Geometry check sheet. Reference: the model listing, model coordinates, mm. A direction names the side the tool comes from. Coordinates: 2 decimals unless noted, no trailing zeros. Loops run counter-clockwise (first coordinate to the right, second up) from the corner with the lowest first, then second, coordinate; pieces in that order, holes last.
Autodesk Inventor part; units mm, degrees
ref_plane "Work Plane1" through (0, 0, 0) normal (0, 0, 1) x (1, 0, 0)
ref_plane "Work Plane2" through (0, 0, 0) normal (0, 0, 1) x (1, 0, 0)
ref_plane "YZ Plane" through (0, 0, 0) normal (1, 0, 0) x (0, 1, 0)
ref_plane "Work Plane1" through (0, 0, 0) normal (0, 0, 1) x (1, 0, 0)
sketch "Sketch1" plane through (0, 0, 0) normal (0, 0, 1) x (1, 0, 0)
  circle A0 centre (0, -92.5) radius 4
  circle A1 centre (0, -102.5) radius 1.5
  circle A2 centre (-10, -92.5) radius 1.5
  circle A3 centre (0, -82.5) radius 1.5
  circle A4 centre (10, -92.5) radius 1.5
  circle A5 centre (0, -92.5) radius 13
  circle A6 centre (0, -92.5) radius 7
  point P0 (0, 0)
  dimension "d0" = 26
  dimension "d1" = 14
extrude "Extrusion1" add sketch "Sketch1" along normal blind 2 contours A5
ref_plane "Work Plane2" through (0, 0, 0) normal (0, 0, 1) x (1, 0, 0)
sketch "Sketch2" plane through (0, 0, 0) normal (0, 0, 1) x (1, 0, 0)
  circle A0 centre (0, -92.5) radius 7
  circle A1 centre (0, -92.5) radius 4
  point P0 (0, 0)
extrude "Extrusion2" add sketch "Sketch2" along normal blind 12
properties part number "AcopleBrida8mm" material "Aluminio 6061"
(1) Sectioned sample at C-C on z = 1. Record the cut outline in (x, y).
Findings:
outline: circle Ø26 at (0, -92.5); hole circle Ø3 at (-10, -92.5); hole circle Ø8 at (0, -92.5); hole circle Ø3 at (0, -102.5); hole circle Ø3 at (0, -82.5); hole circle Ø3 at (10, -92.5)
(2) Gauge pin test, flat ends, axial feed: pin 1 Ø3 at (x, z) = (-5, 9.5) entering from +Y; pin 2 Ø4 at (x, y) = (10, -92.5) entering from +Z; pin 3 Ø3 at (x, z) = (-6, 9) entering from +Y; pin 4 Ø2.5 at (x, y) = (-10, -92.5) entering from -Z. Record the tip position at first contact, or that the pin passes through.
Findings:
pin 1: stops at y = -86.44
pin 2: stops at z = 2
pin 3: stops at y = -87.14
pin 4: passes through
(3) Sectioned sample at A-A on y = -92.5. Record the cut outline in (x, z).
Findings:
outline: (-13, 0) - (-11.5, 0) - (-11.5, 2) - (-13, 2) - close; (-8.5, 0) - (-4, 0) - (-4, 12) - (-7, 12) - (-7, 2) - (-8.5, 2) - close; (4, 0) - (8.5, 0) - (8.5, 2) - (7, 2) - (7, 12) - (4, 12) - close; (11.5, 0) - (13, 0) - (13, 2) - (11.5, 2) - close
(4) Access from +Z, -Z, +X, -X, +Y, -Y to the whole of each face (thin tool, end or side, straight path). Record for faces 4 (the cylindrical face through (-0.91, -99.44, 6.93)), 5 (the cylindrical face through (10, -94, 1)).
Findings:
face 4: +Z
face 5: +Z, -Z
(5) Scan lines: L1, parallel to Y at x = 0, z = 1.25; L2, parallel to Z at x = -6, y = -82; L3, parallel to X at y = -102.5, z = 0.4. Record each from-to range of solid material in increasing order.
Findings:
L1: y = -105.5 to -104, -101 to -96.5, -88.5 to -84, -81 to -79.5
L2: z = 0 to 2
L3: x = -8.31 to -1.5, 1.5 to 8.31
(6) Draft check along X on faces 1 (the cylindrical face through (-2.82, -79.81, 0.99)), 2 (the flat face through (6, -98, 2)), 3 (the cylindrical face through (-10, -94, 1)). Enter one of: +X half, -X half, draft (parallel to the pull), parting line (faces both ways), or undercut.
Findings:
face 1: parting line
face 2: draft
face 3: undercut
(7) Sectioned sample at D-D on x = 3.5. Record the cut outline in (y, z).
Findings:
outline: (-105.02, 0) - (-94.44, 0) - (-94.44, 12) - (-98.56, 12) - (-98.56, 2) - (-105.02, 2) - close; (-90.56, 0) - (-79.98, 0) - (-79.98, 2) - (-86.44, 2) - (-86.44, 12) - (-90.56, 12) - close
(8) Sectioned sample at B-B on x = 0. Record the cut outline in (y, z).
Findings:
outline: (-105.5, 0) - (-104, 0) - (-104, 2) - (-105.5, 2) - close; (-101, 0) - (-96.5, 0) - (-96.5, 12) - (-99.5, 12) - (-99.5, 2) - (-101, 2) - close; (-88.5, 0) - (-84, 0) - (-84, 2) - (-85.5, 2) - (-85.5, 12) - (-88.5, 12) - close; (-81, 0) - (-79.5, 0) - (-79.5, 2) - (-81, 2) - close
